Work out the finished part from the listing and answer in its coordinate system (mm). A direction names the side the tool comes from. Give positions to 0.01 mm unless a question says otherwise; leave off trailing zeros. Order: outer loops, then holes, each group sorted by start corner. A loop starts at its lowest first (then second) coordinate and runs counter-clockwise, first axis right, second up. Notation, with made-up numbers: M -4,-20.5 L 9,-20.5 A8 cw 9,-14.5 Z; hole C 52,59.25 d3. An arc over 180 degrees is marked long. One line per item, written item: value.
Autodesk Inventor part; units mm, degrees
ref_plane "YZ Plane" through (0, 0, 0) normal (1, 0, 0) x (0, 1, 0)
ref_plane "XZ Plane" through (0, 0, 0) normal (0, 1, 0) x (-1, 0, 0)
ref_plane "XY Plane" through (0, 0, 0) normal (0, 0, 1) x (1, 0, 0)
sketch "Schizzo1" plane through (0, 0, 0) normal (0, 1, 0) x (-1, 0, 0)
  line L0 (-35, 10) -> (35, 10)
  line L1 (35, 10) -> (35, -10)
  line L2 (35, -10) -> (-35, -10)
  line L3 (-35, -10) -> (-35, 10)
  line L4 (-35, 10) -> (35, -10) construction
  line L5 (35, 10) -> (-35, -10) construction
  point P0 (0, 0)
  dimension "d0" = 70
  dimension "d1" = 20
extrude "Estrusione1" add sketch "Schizzo1" along normal blind 4
sketch "Schizzo2" plane through (0, 0, 0) normal (0, -1, 0) x (1, 0, 0)
  line L0 (-31, 0) -> (-35, 0)
  line L1 (-35, 0) -> (-35, 5)
  line L2 (-35, 5) -> (-31, 5)
  line L3 (-31, 5) -> (-31, 0)
  line L4 (-35, -5) -> (-31, -5)
  line L5 (-31, -5) -> (-31, -10)
  line L6 (-31, -10) -> (-35, -10)
  line L7 (-35, -10) -> (-35, -5)
  line L8 (35, 0) -> (31, 0)
  line L9 (31, 0) -> (31, 5)
  line L10 (31, 5) -> (35, 5)
  line L11 (35, 5) -> (35, 0)
  line L12 (31, -5) -> (35, -5)
  line L13 (35, -5) -> (35, -10)
  line L14 (35, -10) -> (31, -10)
  line L15 (31, -10) -> (31, -5)
  point P0 (0, 0)
extrude "Estrusione2" cut sketch "Schizzo2" against normal blind 10
properties part number "sotto"
(1) Section B-B, the plane z = -8.25 is taken. Give the vertices of the cut face in (x, y).
Findings:
outline: M -31,0 L 31,0 L 31,4 L -31,4 Z
(2) Which of the six approach directions +Z, -Z, +X, -X, +Y, -Y give full straight-line access (tool end or side, diameter ignored) to faces 1 (the flat face through (-31, 2, -7)), 2 (the flat face through (33, 2, -5)), 3 (the flat face through (33, 2, 5))?
Findings:
face 1: -Z, -X, +Y, -Y
face 2: -Z, +X, +Y, -Y
face 3: +X, +Y, -Y
(3) Given P1, Ø1.5, axis at x = 16, z = 6.5, coming from the -Y side; P2, Ø1.2, axis at y = 2, z = -6.5, coming from the +X side; P3, Ø2, axis at x = -33, y = 2, coming from the -Z side, each flat-ended and moving along its own axis, determine where each tip first touches the part or whether it passes through.
Findings:
P1: stops at y = 0
P2: stops at x = 31
P3: stops at z = -5
(4) Find the intervals of material crossed by probe 1 along X at (y, z) = (1.15, 0.25), in increasing order. Write a range as from..to.
Findings:
probe 1: x = -31..31
(5) Section A-A, the plane y = 2.1 is taken. Give the vertices of the cut face in (x, z).
Findings:
outline: M -35,-5 L -31,-5 L -31,-10 L 31,-10 L 31,-5 L 35,-5 L 35,0 L 31,0 L 31,5 L 35,5 L 35,10 L -35,10 L -35,5 L -31,5 L -31,0 L -35,0 Z
(6) Determine the mould class of faces 4 (the flat face through (-33, 2, 5)), 5 (the flat face through (0, 4, 0)), 6 (the flat face through (-33, 2, -5)) for opening direction Z: pulls with the +Z half, pulls with the -Z half, needs draft (parallel to the pull), parting line crosses it, or undercut.
Findings:
face 4: undercut
face 5: needs draft
face 6: pulls with the -Z half
